from build123d import *

# Parameters (mm, degrees)
F1_DEPTH = 12.5
F3_DEPTH = 25
F4_R     = 1.25
F5_DEPTH = 25


with BuildPart() as f1:
    # F0 (on Right) → F1 (new body, symmetric)
    with BuildSketch(Plane.YZ):
        with BuildLine():
            Line((-2.746685, 2), (-2.746685, 0))
            Line((-2.746685, 0), (45.253315, 0))
            ThreePointArc((45.253315, 0), (46.667529, 0.585786), (47.253315, 2))
            Line((47.253315, 2), (47.253315, 20))
            Line((47.253315, 20), (45.253315, 20))
            Line((45.253315, 20), (45.253315, 2))
            Line((45.253315, 2), (-2.746685, 2))
        make_face()
    extrude(amount=F1_DEPTH, both=True)

    # F2 (on face) → F3 (cut)
    with BuildSketch(Plane.XZ.offset(-45.253315)):
        with BuildLine():
            Line((4.75, 12.75), (-4.75, 12.75))
            ThreePointArc((-4.75, 12.75), (-7.5, 10), (-4.75, 7.25))
            Line((-4.75, 7.25), (4.75, 7.25))
            ThreePointArc((4.75, 7.25), (7.5, 10), (4.75, 12.75))
        make_face()
    extrude(amount=-F3_DEPTH, mode=Mode.SUBTRACT)

    # F4 (on face) → F5 (cut)
    with BuildSketch(Plane(origin=(0, 0, 0), x_dir=(1, 0, 0), z_dir=(0, 0, -1))):
        with Locations((5.5, -19.253315)):
            Circle(F4_R)
        with Locations((-5.5, -19.253315)):
            Circle(F4_R)
    extrude(amount=-F5_DEPTH, mode=Mode.SUBTRACT)


solid = f1.part
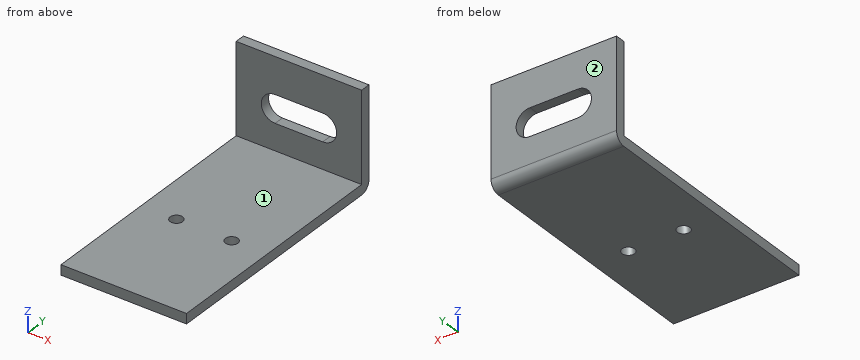
Check sheet for the modelled part. Datum: model origin and axes. Units: mm. Face numbers are marked on the shaded views. A direction names the side the tool comes from. Round coordinates to 2 decimals unless told otherwise and drop trailing zeros. Write each loop counter-clockwise with the first axis right and the second up, starting at its lowest first coordinate (ties: lowest second). Pieces come first, ordered by that corner, then holes. Notation, with made-up numbers: (11, 65.5) - (67, 65.5) arc R21 ccw to (67, 83.5) - close; hole circle Ø9 at (21, 50.25). An arc over 180 degrees is marked (long way). Return JSON: item names as keys, results as strings.
Q1. Access from +Z, -Z, +X, -X, +Y, -Y to the whole of each face (thin tool, end or side, straight path). Record for the marked faces 1 and 2.
Returned:
{"face 1": "+Z, +X, -X, -Y", "face 2": "+Z, -Z, +X, -X, +Y"}
Q2. Cross-section at C-C (x = -8.25). Record the boundary of the cut face in (y, z), then the cut area to 3 significant figures.
Returned:
{"outline": "(-2.75, 0) - (45.25, 0) arc R2 ccw to (47.25, 2) - (47.25, 20) - (45.25, 20) - (45.25, 2) - (-2.75, 2) - close", "area": "135 mm²"}
Q3. Cross-section at A-A (x = -1.75). Record the boundary of the cut face in (y, z), then the cut area to 3 significant figures.
Returned:
{"outline": "(-2.75, 0) - (45.25, 0) arc R2 ccw to (47.25, 2) - (47.25, 7.25) - (45.25, 7.25) - (45.25, 2) - (-2.75, 2) - close; (45.25, 12.75) - (47.25, 12.75) - (47.25, 20) - (45.25, 20) - close", "area": "124 mm²"}
Q4. Cross-section at D-D (x = -5.5). Record the boundary of the cut face in (y, z).
Returned:
{"outline": "(-2.75, 0) - (18, 0) - (18, 2) - (-2.75, 2) - close; (20.5, 0) - (45.25, 0) arc R2 ccw to (47.25, 2) - (47.25, 7.35) - (45.25, 7.35) - (45.25, 2) - (20.5, 2) - close; (45.25, 12.65) - (47.25, 12.65) - (47.25, 20) - (45.25, 20) - close"}
Q5. Scan lines: L1, parallel to Z at x = -2.5, y = 13; L2, parallel to Y at x = -0.25, z = 4; L3, parallel to Y at x = 5.5, z = 1.3. Record each from-to range of solid material in increasing order. Write a range as from..to.
Returned:
{"L1": "z = 0..2", "L2": "y = 45.25..47.25", "L3": "y = -2.75..18, 20.5..47.13"}
Q6. Depth check by flat-ended pin: P1, Ø6, axis at y = 39, z = 3.5, coming from the -X side; P2, Ø4, axis at x = 10, y = 11.5, coming from the +Z side; P3, Ø9, axis at x = -1.5, z = 13, coming from the -Y side. Enter the tip coordinate at first touch or a pass-through.
Returned:
{"P1": "stops at x = -12.5", "P2": "stops at z = 2", "P3": "stops at y = 45.25"}
Q7. Cross-section at B-B (z = 10). Record the boundary of the cut face in (x, y), then the cut area to 3 significant figures.
Returned:
{"outline": "(-12.5, 45.25) - (-7.5, 45.25) - (-7.5, 47.25) - (-12.5, 47.25) - close; (7.5, 45.25) - (12.5, 45.25) - (12.5, 47.25) - (7.5, 47.25) - close", "area": "20.0 mm²"}
